Could you check a few things on this model? Use its own coordinates, in mm. Coordinates: 2 decimals unless noted, no trailing zeros. Order: outer loops, then holes, each group sorted by start corner. A loop starts at its lowest first (then second) coordinate and runs counter-clockwise, first axis right, second up. Notation, with made-up numbers: (22.25, 29) - (76.25, 29) arc R23 cw to (76.25, 55) - close; hole circle Ø6 at (4.25, 36). An arc over 180 degrees is marked (long way). Answer as a JSON object with one key per item and string values. Group by question number.
(1) We'd pull the mould along Y, two halves only. Please class faces 1 (the cylindrical face through (72.16, 246.78, 3.13)), 2 (the cylindrical face through (72.508, 67.264, 3.131)), 3 (the flat face through (175, 159, 0)): pulls with the +Y half, pulls with the -Y half, needs draft (parallel to the pull), parting line crosses it, or undercut.
(2) Imagine slicing it at C-C, the plane z = 5.25. Give the number of separate pieces and of enclosed holes in the cut face, and give its area (3 significant figures).
(3) Please list where these lines run through material, in increasing order: probe 1 along Y at (x, z) = (327.5, 4.5); probe 2 along Y at (x, z) = (74, 2); probe 3 along X at (y, z) = (293, 2).
(4) Imagine slicing it at B-B, the plane x = 304.8. Write out the boundary of the cut face in (y, z), and give its area (3 significant figures).
(5) Will these pins go through, and if not, where does the flat tip stop? P1, Ø3, axis at x = 49, z = 3, coming from the +Y side; P2, Ø3, axis at y = 48, z = 3.5, coming from the -X side.
(6) Imagine slicing it at A-A, the plane x = 50.8. Write out the boundary of the cut face in (y, z).
from build123d import *

# Parameters (mm, degrees)
F0_W     = 19.05
F0_H     = 6.35
F0_R     = 3.96875
F1_DEPTH = 6.35


with BuildPart() as f1:
    # F0 (on Top) → F1 (new body)
    with BuildSketch(Plane.XY):
        with BuildLine():
            Line((0, 309.391197), (0, 4.591197))
            Line((0, 4.591197), (45.640625, 4.591197))
            Line((45.640625, 4.591197), (45.640625, 17.291197))
            ThreePointArc((45.640625, 17.291197), (50.8, 22.450572), (55.959375, 17.291197))
            Line((55.959375, 17.291197), (55.959375, 4.591197))
            Line((55.959375, 4.591197), (299.640625, 4.591197))
            Line((299.640625, 4.591197), (299.640625, 17.291197))
            ThreePointArc((299.640625, 17.291197), (304.8, 22.450572), (309.959375, 17.291197))
            Line((309.959375, 17.291197), (309.959375, 4.591197))
            Line((309.959375, 4.591197), (355.6, 4.591197))
            Line((355.6, 4.591197), (355.6, 309.391197))
            Line((355.6, 309.391197), (309.959375, 309.391197))
            Line((309.959375, 309.391197), (309.959375, 296.691197))
            ThreePointArc((309.959375, 296.691197), (304.8, 291.531822), (299.640625, 296.691197))
            Line((299.640625, 296.691197), (299.640625, 309.391197))
            Line((299.640625, 309.391197), (55.959375, 309.391197))
            Line((55.959375, 309.391197), (55.959375, 296.691197))
            ThreePointArc((55.959375, 296.691197), (50.8, 291.531822), (45.640625, 296.691197))
            Line((45.640625, 296.691197), (45.640625, 309.391197))
            Line((45.640625, 309.391197), (0, 309.391197))
        make_face()
        with Locations((47.625, 47.453697)):
            Rectangle(F0_W, F0_H, mode=Mode.SUBTRACT)
        with Locations((47.625, 79.203697)):
            Rectangle(F0_W, F0_H, mode=Mode.SUBTRACT)
        with Locations((73.025, 63.328697)):
            Circle(F0_R, mode=Mode.SUBTRACT)
        with Locations((187.325, 47.453697)):
            Rectangle(F0_W, F0_H, mode=Mode.SUBTRACT)
        with Locations((187.325, 79.203697)):
            Rectangle(F0_W, F0_H, mode=Mode.SUBTRACT)
        with Locations((327.025, 47.453697)):
            Rectangle(F0_W, F0_H, mode=Mode.SUBTRACT)
        with Locations((327.025, 79.203697)):
            Rectangle(F0_W, F0_H, mode=Mode.SUBTRACT)
        with Locations((333.375, 63.328697)):
            Circle(F0_R, mode=Mode.SUBTRACT)
        with Locations((47.625, 234.778697)):
            Rectangle(F0_W, F0_H, mode=Mode.SUBTRACT)
        with Locations((73.025, 250.653697)):
            Circle(F0_R, mode=Mode.SUBTRACT)
        with Locations((47.625, 266.528697)):
            Rectangle(F0_W, F0_H, mode=Mode.SUBTRACT)
        with Locations((187.325, 234.778697)):
            Rectangle(F0_W, F0_H, mode=Mode.SUBTRACT)
        with Locations((187.325, 266.528697)):
            Rectangle(F0_W, F0_H, mode=Mode.SUBTRACT)
        with Locations((327.025, 234.778697)):
            Rectangle(F0_W, F0_H, mode=Mode.SUBTRACT)
        with Locations((333.375, 250.653697)):
            Circle(F0_R, mode=Mode.SUBTRACT)
        with Locations((327.025, 266.528697)):
            Rectangle(F0_W, F0_H, mode=Mode.SUBTRACT)
    extrude(amount=F1_DEPTH)


solid = f1.part
Result set:
{
 "1": {"face 1": "undercut", "face 2": "undercut", "face 3": "needs draft"},
 "2": {"separate pieces": "1", "enclosed holes": "16", "area": "106,000 mm^2"},
 "3": {"probe 1": "y = 4.59 to 44.28, 50.63 to 76.03, 82.38 to 231.6, 237.95 to 263.35, 269.7 to 309.39", "probe 2": "y = 4.59 to 59.48, 67.18 to 246.81, 254.5 to 309.39", "probe 3": "x = 0 to 47.2, 54.4 to 301.2, 308.4 to 355.6"},
 "4": {"outline": "(22.45, 0) - (291.53, 0) - (291.53, 6.35) - (22.45, 6.35) - close", "area": "1,710 mm^2"},
 "5": {"P1": "stops at y = 292.73", "P2": "stops at x = 0"},
 "6": {"outline": "(22.45, 0) - (44.28, 0) - (44.28, 6.35) - (22.45, 6.35) - close; (50.63, 0) - (76.03, 0) - (76.03, 6.35) - (50.63, 6.35) - close; (82.38, 0) - (231.6, 0) - (231.6, 6.35) - (82.38, 6.35) - close; (237.95, 0) - (263.35, 0) - (263.35, 6.35) - (237.95, 6.35) - close; (269.7, 0) - (291.53, 0) - (291.53, 6.35) - (269.7, 6.35) - close"}
}
